Solid Edge part; units mm, degrees
sketch "Sketch1" plane through (0, 0, 0) normal (0, 0, 1) x (1, 0, 0)
  circle A0 centre (0, 0) radius 6.5
  circle A1 centre (0, 0) radius 7.5
extrude "Protrusion1" add sketch "Sketch1" along normal blind 15
sketch "Sketch2" plane through (0, 0, 15) normal (0, 0, 1) x (1, 0, 0)
  line L0 (0, 7.4) -> (6, 7.4)
  line L1 (6, 7.4) -> (6, 8.4)
  line L2 (6, 8.4) -> (-6, 8.4)
  line L3 (-6, 8.4) -> (-6, 7.4)
  line L4 (-6, 7.4) -> (0, 7.4)
extrude "ExtrudedProtrusion_2" add sketch "Sketch2" along normal blind 8 and the other way blind 1
sketch "Sketch3" plane through (0, 7.4, 18.5) normal (0, -1, 0) x (-1, 0, 0)
  line L0 (-6, 4.5) -> (6, 4.5)
  line L1 (6, 4.5) -> (6, 3.5)
  line L2 (6, 3.5) -> (-6, 3.5)
  line L3 (-6, 4.5) -> (-6, 3.5)
extrude "Protrusion2" add sketch "Sketch3" along normal up to next
extrude "Cutout1" [suppressed]
properties material "Copper"
Check sheet for the modelled part. Datum: model origin and axes. Units: mm. A direction names the side the tool comes from. Give positions to 0.01 mm unless a question says otherwise; leave off trailing zeros. Loops run counter-clockwise (first coordinate to the right, second up) from the corner with the lowest first, then second, coordinate; pieces in that order, holes last. Notation, with made-up numbers: M 49,17.5 L 59,17.5 A15 cw 59,28.5 Z; hole C 74,-6 d3. An arc over 180 degrees is marked long. Return JSON: item names as keys, results as strings. Group by question number.
1. Tool access check on faces 5 (the flat face through (6, 8, 18)), 6 (the flat face through (0, 8, 14)), 7 (the flat face through (0, 7, 15)), 8 (the flat face through (-6, 3, 0)), 9 (the flat face through (0, 8.4, 18)). Record the directions out of +Z, -Z, +X, -X, +Y, -Y that give a thin tool (end or side, any length) a straight path to the whole face; none if there is none.
2. Thickness scan on L1, parallel to Y at x = 0.25, z = 13.25; L2, parallel to X at y = 2, z = 10.75; L3, parallel to Y at x = -5, z = 18.5. Record the ranges inside material, lowest first.
3. Cross-section at A-A on y = 0. Record the boundary of the cut face in (x, z).
4. Mould release check, pull along Y, two halves, no side actions. Record for faces 1 (the flat face through (0, 7.4, 19)), 2 (the flat face through (-6, 8, 18)), 3 (the cylindrical face through (-5.158, 3.955, 7.395)), 4 (the cylindrical face through (-0.976, -7.436, 7.395)): released by +Y, released by -Y, zero draft, split by the parting line, or undercut.
5. Cross-section at D-D on y = 5.5. Record the boundary of the cut face in (x, z), plus the area to 3 significant figures.
6. Cross-section at B-B on x = 0. Record the boundary of the cut face in (y, z).
7. Go/stop test with flat-tipped pins: pin 1 (2 mm diameter, centred on y = 6.5, z = 19, fed in from -X); pin 2 (8 mm diameter, centred on x = -5, y = 3, fed in from +Z); pin 3 (6 mm diameter, centred on y = -4.5, z = 9.5, fed in from +X); pin 4 (4.5 mm diameter, centred on x = 0, y = 6.5, fed in from -Z). Record where each tip stops, or that it passes through.
8. Cross-section at C-C on z = 17.25. Record the boundary of the cut face in (x, y).
Return value:
{
 "1": {"face 5": "+Z, -Z, +X, +Y", "face 6": "-Z, +Y", "face 7": "+Z, +X, -X, -Y", "face 8": "-Z, +X, -X, +Y, -Y", "face 9": "+Z, -Z, +X, -X, +Y"},
 "2": {"L1": "-7.5 to -6.5, 6.5 to 7.5", "L2": "-7.23 to -6.18, 6.18 to 7.23", "L3": "7.4 to 8.4"},
 "3": {"outline": "M -7.5,0 L -6.5,0 L -6.5,15 L -7.5,15 Z; M 6.5,0 L 7.5,0 L 7.5,15 L 6.5,15 Z"},
 "4": {"face 1": "released by -Y", "face 2": "zero draft", "face 3": "undercut", "face 4": "split by the parting line"},
 "5": {"outline": "M -6,14 L -5.1,14 L -5.1,0 L -3.46,0 L -3.46,15 L -6,15 Z; M 3.46,0 L 5.1,0 L 5.1,14 L 6,14 L 6,15 L 3.46,15 Z", "area": "50.8 mm^2"},
 "6": {"outline": "M -7.5,0 L -6.5,0 L -6.5,15 L -7.5,15 Z; M 6.5,0 L 7.5,0 L 7.5,14 L 8.4,14 L 8.4,23 L 7.4,23 L 7.4,15 L 6.5,15 Z"},
 "7": {"pin 1": "x = -6", "pin 2": "z = 15", "pin 3": "x = 7.35", "pin 4": "z = 0"},
 "8": {"outline": "M -6,7.4 L 6,7.4 L 6,8.4 L -6,8.4 Z"}
}
